from build123d import *

# Parameters (mm, degrees)
F1_DEPTH  = 25
F2_R      = 90
F3_DEPTH  = 5
F4_R      = 30
F4_R_2    = 15
F5_DEPTH  = 30
F5_FACE_R = 15
F6_DEPTH  = 100
F7_SIZE   = 4


with BuildPart() as f1:
    # F0 (on Front) → F1 (new body)
    with BuildSketch(Plane.XZ):
        with BuildLine():
            ThreePointArc((99.499436, -9.99311), (99.874781, -5.002819), (100, 0))
            ThreePointArc((100, 0), (99.874781, 5.002819), (99.499436, 9.99311))
            ThreePointArc((99.499436, 9.99311), (98.768834, 15.643447), (97.717628, 21.243005))
            ThreePointArc((97.717628, 21.243005), (95.105652, 30.901699), (91.541546, 40.251029))
            ThreePointArc((91.541546, 40.251029), (89.100652, 45.39905), (86.370537, 50.399706))
            ThreePointArc((86.370537, 50.399706), (80.901699, 58.778525), (74.622932, 66.568897))
            ThreePointArc((74.622932, 66.568897), (70.710678, 70.710678), (66.568897, 74.622932))
            ThreePointArc((66.568897, 74.622932), (58.778525, 80.901699), (50.399706, 86.370537))
            ThreePointArc((50.399706, 86.370537), (45.39905, 89.100652), (40.251029, 91.541546))
            ThreePointArc((40.251029, 91.541546), (30.901699, 95.105652), (21.243005, 97.717628))
            ThreePointArc((21.243005, 97.717628), (15.643447, 98.768834), (9.99311, 99.499436))
            ThreePointArc((9.99311, 99.499436), (0, 100), (-9.99311, 99.499436))
            ThreePointArc((-9.99311, 99.499436), (-15.643447, 98.768834), (-21.243005, 97.717628))
            ThreePointArc((-21.243005, 97.717628), (-30.901699, 95.105652), (-40.251029, 91.541546))
            ThreePointArc((-40.251029, 91.541546), (-45.39905, 89.100652), (-50.399706, 86.370537))
            ThreePointArc((-50.399706, 86.370537), (-58.778525, 80.901699), (-66.568897, 74.622932))
            ThreePointArc((-66.568897, 74.622932), (-70.710678, 70.710678), (-74.622932, 66.568897))
            ThreePointArc((-74.622932, 66.568897), (-80.901699, 58.778525), (-86.370537, 50.399706))
            ThreePointArc((-86.370537, 50.399706), (-89.100652, 45.39905), (-91.541546, 40.251029))
            ThreePointArc((-91.541546, 40.251029), (-95.105652, 30.901699), (-97.717628, 21.243005))
            ThreePointArc((-97.717628, 21.243005), (-98.768834, 15.643447), (-99.499436, 9.99311))
            ThreePointArc((-99.499436, 9.99311), (-100, 0), (-99.499436, -9.99311))
            ThreePointArc((-99.499436, -9.99311), (-98.768834, -15.643447), (-97.717628, -21.243005))
            ThreePointArc((-97.717628, -21.243005), (-95.105652, -30.901699), (-91.541546, -40.251029))
            ThreePointArc((-91.541546, -40.251029), (-89.100652, -45.39905), (-86.370537, -50.399706))
            ThreePointArc((-86.370537, -50.399706), (-80.901699, -58.778525), (-74.622932, -66.568897))
            ThreePointArc((-74.622932, -66.568897), (-70.710678, -70.710678), (-66.568897, -74.622932))
            ThreePointArc((-66.568897, -74.622932), (-58.778525, -80.901699), (-50.399706, -86.370537))
            ThreePointArc((-50.399706, -86.370537), (-45.39905, -89.100652), (-40.251029, -91.541546))
            ThreePointArc((-40.251029, -91.541546), (-30.901699, -95.105652), (-21.243005, -97.717628))
            ThreePointArc((-21.243005, -97.717628), (-15.643447, -98.768834), (-9.99311, -99.499436))
            ThreePointArc((-9.99311, -99.499436), (0, -100), (9.99311, -99.499436))
            ThreePointArc((9.99311, -99.499436), (15.643447, -98.768834), (21.243005, -97.717628))
            ThreePointArc((21.243005, -97.717628), (30.901699, -95.105652), (40.251029, -91.541546))
            ThreePointArc((40.251029, -91.541546), (45.39905, -89.100652), (50.399706, -86.370537))
            ThreePointArc((50.399706, -86.370537), (58.778525, -80.901699), (66.568897, -74.622932))
            ThreePointArc((66.568897, -74.622932), (70.710678, -70.710678), (74.622932, -66.568897))
            ThreePointArc((74.622932, -66.568897), (80.901699, -58.778525), (86.370537, -50.399706))
            ThreePointArc((86.370537, -50.399706), (89.100652, -45.39905), (91.541546, -40.251029))
            ThreePointArc((91.541546, -40.251029), (95.105652, -30.901699), (97.717628, -21.243005))
            ThreePointArc((97.717628, -21.243005), (98.768834, -15.643447), (99.499436, -9.99311))
        make_face()
        with BuildLine():
            ThreePointArc((-99.499436, -9.99311), (-100, 0), (-99.499436, 9.99311))
            Line((-99.499436, 9.99311), (-120, 4.5))
            Line((-120, 4.5), (-120, 0))
            Line((-120, 0), (-120, -4.5))
            Line((-120, -4.5), (-99.499436, -9.99311))
        make_face()
        with BuildLine():
            ThreePointArc((-97.717628, 21.243005), (-95.105652, 30.901699), (-91.541546, 40.251029))
            Line((-91.541546, 40.251029), (-112.736205, 41.361794))
            Line((-112.736205, 41.361794), (-114.126782, 37.082039))
            Line((-114.126782, 37.082039), (-115.517358, 32.802285))
            Line((-115.517358, 32.802285), (-97.717628, 21.243005))
        make_face()
        with BuildLine():
            ThreePointArc((-86.370537, 50.399706), (-80.901699, 58.778525), (-74.622932, 66.568897))
            Line((-74.622932, 66.568897), (-94.437006, 74.174807))
            Line((-94.437006, 74.174807), (-97.082039, 70.53423))
            Line((-97.082039, 70.53423), (-99.727073, 66.893654))
            Line((-99.727073, 66.893654), (-86.370537, 50.399706))
        make_face()
        with BuildLine():
            ThreePointArc((-66.568897, 74.622932), (-58.778525, 80.901699), (-50.399706, 86.370537))
            Line((-50.399706, 86.370537), (-66.893654, 99.727073))
            Line((-66.893654, 99.727073), (-70.53423, 97.082039))
            Line((-70.53423, 97.082039), (-74.174807, 94.437006))
            Line((-74.174807, 94.437006), (-66.568897, 74.622932))
        make_face()
        with BuildLine():
            ThreePointArc((-40.251029, 91.541546), (-30.901699, 95.105652), (-21.243005, 97.717628))
            Line((-21.243005, 97.717628), (-32.802285, 115.517358))
            Line((-32.802285, 115.517358), (-37.082039, 114.126782))
            Line((-37.082039, 114.126782), (-41.361794, 112.736205))
            Line((-41.361794, 112.736205), (-40.251029, 91.541546))
        make_face()
        with BuildLine():
            ThreePointArc((-9.99311, 99.499436), (0, 100), (9.99311, 99.499436))
            Line((9.99311, 99.499436), (4.5, 120))
            Line((4.5, 120), (0, 120))
            Line((0, 120), (-4.5, 120))
            Line((-4.5, 120), (-9.99311, 99.499436))
        make_face()
        with BuildLine():
            ThreePointArc((21.243005, 97.717628), (30.901699, 95.105652), (40.251029, 91.541546))
            Line((40.251029, 91.541546), (41.361794, 112.736205))
            Line((41.361794, 112.736205), (37.082039, 114.126782))
            Line((37.082039, 114.126782), (32.802285, 115.517358))
            Line((32.802285, 115.517358), (21.243005, 97.717628))
        make_face()
        with BuildLine():
            ThreePointArc((50.399706, 86.370537), (58.778525, 80.901699), (66.568897, 74.622932))
            Line((66.568897, 74.622932), (74.174807, 94.437006))
            Line((74.174807, 94.437006), (70.53423, 97.082039))
            Line((70.53423, 97.082039), (66.893654, 99.727073))
            Line((66.893654, 99.727073), (50.399706, 86.370537))
        make_face()
        with BuildLine():
            ThreePointArc((74.622932, 66.568897), (80.901699, 58.778525), (86.370537, 50.399706))
            Line((86.370537, 50.399706), (99.727073, 66.893654))
            Line((99.727073, 66.893654), (97.082039, 70.53423))
            Line((97.082039, 70.53423), (94.437006, 74.174807))
            Line((94.437006, 74.174807), (74.622932, 66.568897))
        make_face()
        with BuildLine():
            ThreePointArc((91.541546, 40.251029), (95.105652, 30.901699), (97.717628, 21.243005))
            Line((97.717628, 21.243005), (115.517358, 32.802285))
            Line((115.517358, 32.802285), (114.126782, 37.082039))
            Line((114.126782, 37.082039), (112.736205, 41.361794))
            Line((112.736205, 41.361794), (91.541546, 40.251029))
        make_face()
        with BuildLine():
            ThreePointArc((99.499436, 9.99311), (99.874781, 5.002819), (100, 0))
            ThreePointArc((100, 0), (99.874781, -5.002819), (99.499436, -9.99311))
            Line((99.499436, -9.99311), (120, -4.5))
            Line((120, -4.5), (120, 0))
            Line((120, 0), (120, 4.5))
            Line((120, 4.5), (99.499436, 9.99311))
        make_face()
        with BuildLine():
            Line((115.517358, -32.802285), (97.717628, -21.243005))
            ThreePointArc((97.717628, -21.243005), (95.105652, -30.901699), (91.541546, -40.251029))
            Line((91.541546, -40.251029), (112.736205, -41.361794))
            Line((112.736205, -41.361794), (114.126782, -37.082039))
            Line((114.126782, -37.082039), (115.517358, -32.802285))
        make_face()
        with BuildLine():
            Line((99.727073, -66.893654), (86.370537, -50.399706))
            ThreePointArc((86.370537, -50.399706), (80.901699, -58.778525), (74.622932, -66.568897))
            Line((74.622932, -66.568897), (94.437006, -74.174807))
            Line((94.437006, -74.174807), (97.082039, -70.53423))
            Line((97.082039, -70.53423), (99.727073, -66.893654))
        make_face()
        with BuildLine():
            Line((74.174807, -94.437006), (66.568897, -74.622932))
            ThreePointArc((66.568897, -74.622932), (58.778525, -80.901699), (50.399706, -86.370537))
            Line((50.399706, -86.370537), (66.893654, -99.727073))
            Line((66.893654, -99.727073), (70.53423, -97.082039))
            Line((70.53423, -97.082039), (74.174807, -94.437006))
        make_face()
        with BuildLine():
            Line((41.361794, -112.736205), (40.251029, -91.541546))
            ThreePointArc((40.251029, -91.541546), (30.901699, -95.105652), (21.243005, -97.717628))
            Line((21.243005, -97.717628), (32.802285, -115.517358))
            Line((32.802285, -115.517358), (37.082039, -114.126782))
            Line((37.082039, -114.126782), (41.361794, -112.736205))
        make_face()
        with BuildLine():
            Line((4.5, -120), (9.99311, -99.499436))
            ThreePointArc((9.99311, -99.499436), (0, -100), (-9.99311, -99.499436))
            Line((-9.99311, -99.499436), (-4.5, -120))
            Line((-4.5, -120), (0, -120))
            Line((0, -120), (4.5, -120))
        make_face()
        with BuildLine():
            Line((-32.802285, -115.517358), (-21.243005, -97.717628))
            ThreePointArc((-21.243005, -97.717628), (-30.901699, -95.105652), (-40.251029, -91.541546))
            Line((-40.251029, -91.541546), (-41.361794, -112.736205))
            Line((-41.361794, -112.736205), (-37.082039, -114.126782))
            Line((-37.082039, -114.126782), (-32.802285, -115.517358))
        make_face()
        with BuildLine():
            Line((-66.893654, -99.727073), (-50.399706, -86.370537))
            ThreePointArc((-50.399706, -86.370537), (-58.778525, -80.901699), (-66.568897, -74.622932))
            Line((-66.568897, -74.622932), (-74.174807, -94.437006))
            Line((-74.174807, -94.437006), (-70.53423, -97.082039))
            Line((-70.53423, -97.082039), (-66.893654, -99.727073))
        make_face()
        with BuildLine():
            Line((-94.437006, -74.174807), (-74.622932, -66.568897))
            ThreePointArc((-74.622932, -66.568897), (-80.901699, -58.778525), (-86.370537, -50.399706))
            Line((-86.370537, -50.399706), (-99.727073, -66.893654))
            Line((-99.727073, -66.893654), (-97.082039, -70.53423))
            Line((-97.082039, -70.53423), (-94.437006, -74.174807))
        make_face()
        with BuildLine():
            Line((-112.736205, -41.361794), (-91.541546, -40.251029))
            ThreePointArc((-91.541546, -40.251029), (-95.105652, -30.901699), (-97.717628, -21.243005))
            Line((-97.717628, -21.243005), (-115.517358, -32.802285))
            Line((-115.517358, -32.802285), (-114.126782, -37.082039))
            Line((-114.126782, -37.082039), (-112.736205, -41.361794))
        make_face()
    extrude(amount=F1_DEPTH)

    # F2 (on face) → F3 (cut)
    with BuildSketch(Plane.XZ.offset(25)):
        Circle(F2_R)
    extrude(amount=-F3_DEPTH, mode=Mode.SUBTRACT)

    # F4 (on face) → F5 (join)
    with BuildSketch(Plane.XZ.offset(20)):
        Circle(F4_R)
        Circle(F4_R_2, mode=Mode.SUBTRACT)
    extrude(amount=F5_DEPTH)

    # F5_face (on face) → F6 (cut)
    with BuildSketch(Plane.XZ.offset(20)):
        Circle(F5_FACE_R)
    extrude(amount=-F6_DEPTH, mode=Mode.SUBTRACT)

    # F7
    f7_edges = [f1.edges().sort_by_distance(p)[0] for p in [
        (-30, -50, 0),
        (-15, -50, 0),
    ]]
    chamfer(f7_edges, length=F7_SIZE)


solid = f1.part
Design review of the part built by this model. Coordinates are the model's own, in mm. A direction names the side the tool comes from. Coordinates: 2 decimals unless noted, no trailing zeros. Order: outer loops, then holes, each group sorted by start corner. A loop starts at its lowest first (then second) coordinate and runs counter-clockwise, first axis right, second up. Notation, with made-up numbers: M -21.5,69 L -10.5,69 A18 ccw -10.5,78 Z; hole C 35,74.25 d3. An arc over 180 degrees is marked long. Use a Markdown table: item, result.
(1) Add section B-B (z = 0). Give the boundary of the cut face in (x, y).
Worked answers:
| item | result |
|---|---|
| outline | M -120,-25 L -90,-25 L -90,-20 L -30,-20 L -30,-46 L -26,-50 L -19,-50 L -15,-46 L -15,0 L -120,0 Z; M 15,-46 L 19,-50 L 26,-50 L 30,-46 L 30,-20 L 90,-20 L 90,-25 L 120,-25 L 120,0 L 15,0 Z |
(2) Wall thickness on probe 1 along Z at (x, y) = (0, -23.65); probe 2 along Z at (x, y) = (0, -30); probe 3 along Z at (x, y) = (101, -5): over which ranges is each line inside the solid? List them lowest first.
Worked answers:
| item | result |
|---|---|
| probe 1 | z = -120 to -90, -30 to -15, 15 to 30, 90 to 120 |
| probe 2 | z = -30 to -15, 15 to 30 |
| probe 3 | z = -40.75 to -23.37, -9.59 to 9.59, 23.37 to 40.75 |
(3) For faces 1 (the flat face through (-92.955, -12.325, -58.531)), 2 (the cylindrical face through (98.756, -12.325, -15.722)), 3 (the cylindrical face through (-15.722, -12.325, -98.756)), 4 (the cylindrical face through (-15.56, -12.32, 98.78)), list the 3-axis set-ups (+Z, -Z, +X, -X, +Y, -Y) from which the entire face can be reached by the end or side of a thin tool; tool diameter is ignored.
Worked answers:
| item | result |
|---|---|
| face 1 | -X, +Y, -Y |
| face 2 | +X, +Y, -Y |
| face 3 | -Z, +Y, -Y |
| face 4 | +Z, +Y, -Y |
(4) Add section A-A (x = 0). Give the boundary of the cut face in (y, z).
Worked answers:
| item | result |
|---|---|
| outline | M -50,-26 L -46,-30 L -20,-30 L -20,-90 L -25,-90 L -25,-120 L 0,-120 L 0,-15 L -46,-15 L -50,-19 Z; M -50,19 L -46,15 L 0,15 L 0,120 L -25,120 L -25,90 L -20,90 L -20,30 L -46,30 L -50,26 Z |
(5) Add section C-C (x = 103.5). Give the boundary of the cut face in (y, z).
Worked answers:
| item | result |
|---|---|
| outline | M -25,-40.88 L 0,-40.88 L 0,-25 L -25,-25 Z; M -25,-8.92 L 0,-8.92 L 0,8.92 L -25,8.92 Z; M -25,25 L 0,25 L 0,40.88 L -25,40.88 Z |
(6) For P1, Ø6, axis at y = -29, z = -2, coming from the +X side; P2, Ø4, axis at x = -54, z = -34.5, coming from the -Y side; P3, Ø4, axis at x = -22, z = 18.5, coming from the -Y side; P4, Ø18, axis at x = 0, z = 0, coming from the -Y side, all flat-tipped, find the tip position at first contact; note any pin that passes through.
Worked answers:
| item | result |
|---|---|
| P1 | stops at x = 30 |
| P2 | stops at y = -20 |
| P3 | stops at y = -49.26 |
| P4 | passes through |
(7) Add section D-D (z = -103). Give the boundary of the cut face in (x, y), then the cut area to 3 significant figures.
Worked answers:
| item | result |
|---|---|
| outline | M -40.85,-25 L -24.67,-25 L -24.67,0 L -40.85,0 Z; M -9.06,-25 L 9.06,-25 L 9.06,0 L -9.06,0 Z; M 24.67,-25 L 40.85,-25 L 40.85,0 L 24.67,0 Z |
| area | 1,260 mm2 |
(8) Draft analysis for pull direction Z (two halves, no side actions). For faces 5 (the cylindrical face through (-89.064, -12.325, 45.47)), 6 (the flat face through (27.1, -12.32, 106.74)), 7 (the flat face through (-106.74, -12.32, 27.1)), 8 (the flat face through (7.21, -12.32, -109.89)), state which applies: released by +Z, released by -Z, zero draft, split by the parting line, or undercut.
Worked answers:
| item | result |
|---|---|
| face 5 | undercut |
| face 6 | released by +Z |
| face 7 | undercut |
| face 8 | released by -Z |
